CAD build for the part. Positions are in the model's coordinates, mm. Round coordinates to 2 decimals unless told otherwise and drop trailing zeros. Loops run counter-clockwise (first coordinate to the right, second up) from the corner with the lowest first, then second, coordinate; pieces in that order, holes last.
```python
from build123d import *

# Parameters (mm, degrees)
SKETCH1_W           = 114
SKETCH1_H           = 40
SKETCH1_R           = 7.45
SKETCH1_R_2         = 9.525
BOSS_EXTRUDE1_DEPTH = 5.08
FILLET1_R           = 10
SKETCH2_R           = 3.175
CUT_EXTRUDE1_DEPTH  = 6.08


with BuildPart() as part:
    # Sketch1 → Boss-Extrude1 (new body)
    with BuildSketch(Plane(origin=(0, 0, 0), x_dir=(1, 0, 0), z_dir=(0, 1, 0))):
        Rectangle(SKETCH1_W, SKETCH1_H)
        with Locations((-45, 0)):
            Circle(SKETCH1_R, mode=Mode.SUBTRACT)
        with Locations((45, 0)):
            Circle(SKETCH1_R, mode=Mode.SUBTRACT)
        Circle(SKETCH1_R_2, mode=Mode.SUBTRACT)
    extrude(amount=BOSS_EXTRUDE1_DEPTH)

    # Fillet1
    fillet1_edges = [part.edges().sort_by_distance(p)[0] for p in [
        (-57, 2.54, -20),
        (57, 2.54, -20),
        (57, 2.54, 20),
        (-57, 2.54, 20),
    ]]
    fillet(fillet1_edges, radius=FILLET1_R)

    # Sketch2 → Cut-Extrude1 (cut, through all)
    with BuildSketch(Plane(origin=(0, 5.08, 0), x_dir=(1, 0, 0), z_dir=(0, 1, 0))):
        with Locations((-10.75, -10.75)):
            Circle(SKETCH2_R)
        with Locations((-10.75, 10.75)):
            Circle(SKETCH2_R)
        with Locations((10.75, 10.75)):
            Circle(SKETCH2_R)
        with Locations((10.75, -10.75)):
            Circle(SKETCH2_R)
    extrude(amount=-CUT_EXTRUDE1_DEPTH, mode=Mode.SUBTRACT)


solid = part.part
```
Item 1: Two-plate mould, pull along X, no slides. Class faces 1 (the cylindrical face through (12.215, 2.576, 13.567)), 2 (the flat face through (-1, 3, 20)), 3 (the flat face through (-57, 3, 0)): released by +X, released by -X, zero draft, split by the parting line, or undercut.
Answers follow:
face 1: undercut
face 2: zero draft
face 3: released by -X
Item 2: Flat gauge pins, fed straight in: P1, Ø5, axis at x = 10.75, z = 10.75, coming from the -Y side; P2, Ø1, axis at y = 4, z = 15, coming from the +X side. Where does each tip first touch, or does it go through?
Answers follow:
P1: passes through
P2: stops at x = 55.93
Item 3: Cut at D-D, the plane z = -1.5. Give the cut face in (x, y).
Answers follow:
outline: (-57, 0) - (-52.3, 0) - (-52.3, 5.08) - (-57, 5.08) - close; (-37.7, 0) - (-9.41, 0) - (-9.41, 5.08) - (-37.7, 5.08) - close; (9.41, 0) - (37.7, 0) - (37.7, 5.08) - (9.41, 5.08) - close; (52.3, 0) - (57, 0) - (57, 5.08) - (52.3, 5.08) - close
Item 4: Cut at C-C, the plane x = -45. Give the cut face in (y, z), plus the area to 3 significant figures.
Answers follow:
outline: (0, -20) - (5.08, -20) - (5.08, -7.45) - (0, -7.45) - close; (0, 7.45) - (5.08, 7.45) - (5.08, 20) - (0, 20) - close
area: 128 mm2
Item 5: Probe line 1 (Z direction, x = -10.75, y = 1.15) (3 decimals); line 2 (X direction, y = 3.8, z = -8); line 3 (X direction, y = 2.1, z = -10.75) (3 decimals). List the from-to ranges inside material, lowest first.
Answers follow:
line 1: z = -20 to -13.925, -7.575 to 7.575, 13.925 to 20
line 2: x = -57 to -12.34, -9.16 to -5.17, 5.17 to 9.16, 12.34 to 57
line 3: x = -56.972 to -13.925, -7.575 to 7.575, 13.925 to 56.972
Item 6: Cut at A-A, the plane x = -10.75. Give the cut face in (y, z) (3 decimals), plus the area to 3 significant figures.
Answers follow:
outline: (0, -20) - (5.08, -20) - (5.08, -13.925) - (0, -13.925) - close; (0, -7.575) - (5.08, -7.575) - (5.08, 7.575) - (0, 7.575) - close; (0, 13.925) - (5.08, 13.925) - (5.08, 20) - (0, 20) - close
area: 139 mm2
Item 7: Cut at B-B, the plane y = 1.6. Give the cut face in (x, z) (3 decimals).
Answers follow:
outline: (-57, -10) arc R10 ccw to (-47, -20) - (47, -20) arc R10 ccw to (57, -10) - (57, 10) arc R10 ccw to (47, 20) - (-47, 20) arc R10 ccw to (-57, 10) - close; hole circle Ø14.9 at (-45, 0); hole circle Ø6.35 at (-10.75, -10.75); hole circle Ø6.35 at (-10.75, 10.75); hole circle Ø19.05 at (0, 0); hole circle Ø6.35 at (10.75, -10.75); hole circle Ø6.35 at (10.75, 10.75); hole circle Ø14.9 at (45, 0)
